from build123d import *

# Parameters (mm, degrees)
EXTRU_MINCE1_DEPTH      = 3
EXTRU_MINCE1_2_DEPTH    = 3
EXTRU_MINCE1_3_DEPTH    = 3
BOSS_EXTRU_1_DEPTH      = 0.25
BOSS_EXTRU_1_DEPTH_BACK = 1
ESQUISSE3_R             = 4.3
ESQUISSE3_R_2           = 0.05
ESQUISSE4_W             = 1.75
ESQUISSE4_H             = 3
EXTRU_MINCE2_DEPTH      = 45
CONG_1_R                = 0.2
ESQUISSE6_R             = 6.8
BOSS_EXTRU_2_DEPTH      = 1.3


# Read off the part's stored shape, not the designer's step: Extru.-Mince2
with BuildPart() as part:
    # Esquisse2 → Extru.-Mince1 (new body)
    with BuildSketch(Plane.XY):
        with BuildLine():
            ThreePointArc((0, 4.2), (2.89149518, 3.046187063), (4.194302481, 0.218693153))
            Line((4.194302481, 0.218693153), (0.049932172, 0.00260349))
            ThreePointArc((0.049932172, 0.00260349), (0.034422562, 0.036264132), (0, 0.05))
            Line((0, 0.05), (0, 4.2))
        make_face()
    extrude(amount=EXTRU_MINCE1_DEPTH)



with BuildPart() as body_2:
    # Esquisse2 → Extru.-Mince1 2 (new body)
    with BuildSketch(Plane.XY):
        with BuildLine():
            ThreePointArc((3.637306696, -2.1), (1.192327791, -4.027201813), (-1.907757414, -3.741719077))
            Line((-1.907757414, -3.741719077), (-0.022711398, -0.044544275))
            ThreePointArc((-0.022711398, -0.044544275), (0.014194378, -0.047942879), (0.04330127, -0.025))
            Line((0.04330127, -0.025), (3.637306696, -2.1))
        make_face()
    extrude(amount=EXTRU_MINCE1_2_DEPTH)


with BuildPart() as body_3:
    # Esquisse2 → Extru.-Mince1 3 (new body)
    with BuildSketch(Plane.XY):
        with BuildLine():
            ThreePointArc((-3.637306696, -2.1), (-4.083822971, 0.98101475), (-2.286545067, 3.523025923))
            Line((-2.286545067, 3.523025923), (-0.027220775, 0.041940785))
            ThreePointArc((-0.027220775, 0.041940785), (-0.04861694, 0.011678747), (-0.04330127, -0.025))
            Line((-0.04330127, -0.025), (-3.637306696, -2.1))
        make_face()
    extrude(amount=EXTRU_MINCE1_3_DEPTH)


with BuildPart() as part_1:
    add(part.part)

    add(body_2.part)  # Boss.-Extru.1 merges body 2

    add(body_3.part)  # Boss.-Extru.1 merges body 3
    # Esquisse3 → Boss.-Extru.1 (add, two sides: drawn at the far end of the back side and taken through both)
    # profile 1 of 2: a face of its own
    with BuildSketch(Plane.XY.offset(-BOSS_EXTRU_1_DEPTH_BACK)):
        Circle(ESQUISSE3_R)
        Circle(ESQUISSE3_R_2, mode=Mode.SUBTRACT)
    # profile 2 of 2: a face of its own
    with BuildSketch(Plane.XY.offset(-BOSS_EXTRU_1_DEPTH_BACK)):
        Circle(ESQUISSE3_R_2)
    extrude(amount=BOSS_EXTRU_1_DEPTH + BOSS_EXTRU_1_DEPTH_BACK)

    # Esquisse4 → Enlèvement de matière-Révolution1 (revolve, cut)
    with BuildSketch(Plane(origin=(0, 0, 0), x_dir=(0, 0, -1), z_dir=(1, 0, 0)), mode=Mode.PRIVATE) as enl_vement_de_mati_re_r_volution1_sk:
        with Locations((-1.625, 2.5)):
            Rectangle(ESQUISSE4_W, ESQUISSE4_H)
    revolve(enl_vement_de_mati_re_r_volution1_sk.sketch.rotate(Axis((0, 0, 0), (0, 0, 1)), 270), axis=Axis((0, 0, 0), (0, 0, 1)), mode=Mode.SUBTRACT)

    # Extru.-Mince2 outline → Extru.-Mince2 (add)
    with BuildSketch(Plane(origin=(0, 0, -1), x_dir=(-1, 0, 0), z_dir=(0, 0, -1))):
        Polygon((0.75, 1.03228644), (0.75, 3.7), (-0.75, 3.7), (-0.75, 1.03228644), (-3.287146365, 1.856655266), (-3.750671856, 0.430070492), (-1.213525492, -0.394298334), (-2.781568179, -2.55252394), (-1.568042688, -3.434201818), (0, -1.275976213), (1.568042688, -3.434201818), (2.781568179, -2.55252394), (1.213525492, -0.394298334), (3.750671856, 0.430070492), (3.287146365, 1.856655266), align=None)
    extrude(amount=EXTRU_MINCE2_DEPTH)

    # Congé1
    cong_1_edges = [part_1.edges().sort_by_distance(p)[0] for p in [
        (1.997546836, -1.473411137, -1),
        (2.018573182, 1.444470853, -1),
        (-2.482098674, 0.017886079, -1),
        (2.482098674, 0.017886079, -1),
        (3.518909111, 1.143362879, -1),
        (0.75, 2.36614322, -1),
        (0, 3.7, -1),
        (-2.018573182, 1.444470853, -1),
        (-3.51890911, 1.143362879, -1),
        (-1.997546836, -1.473411137, -1),
        (-2.174805433, -2.993362879, -1),
        (0.784021344, -2.355089015, -1),
        (2.174805433, -2.993362879, -1),
        (-0.75, 2.36614322, -1),
        (-0.784021344, -2.355089015, -1),
    ]]
    fillet(cong_1_edges, radius=CONG_1_R)

    # Esquisse6 → Boss.-Extru.2 (add)
    with BuildSketch(Plane(origin=(0, 0, -46), x_dir=(-1, 0, 0), z_dir=(0, 0, -1))):
        Circle(ESQUISSE6_R)
    extrude(amount=BOSS_EXTRU_2_DEPTH)


solid = part_1.part
The model under review builds one solid part; all positions refer to its coordinate system, in mm. A direction names the side the tool comes from. Round coordinates to 2 decimals unless told otherwise and drop trailing zeros. Write each loop counter-clockwise with the first axis right and the second up, starting at its lowest first coordinate (ties: lowest second). Pieces come first, ordered by that corner, then holes. Notation, with made-up numbers: (22.25, -18) -> (60.25, -18) arc R31 cw to (60.25, 10) -> close; hole circle Ø6 at (20.25, 43). An arc over 180 degrees is marked (long way). Answer as a JSON object with one key per item and string values.
1. To check wall thickness, follow line 1 along Z through (x, y) = (-5, -1.75); line 2 along X through (y, z) = (2.25, -33.5); line 3 along Y through (x, z) = (-2.25, -5). State the ranges of each line that lie inside material, in increasing order.
Results found:
{"line 1": "z = -47.3 to -46", "line 2": "x = -0.75 to 0.75", "line 3": "y = -2.94 to -1.82, -0.06 to 1.52"}
2. The part is to be moulded in two halves that separate along Z. For faces 1 (the face through (-3, 1, 3)), 2 (the face through (2.859, 3.077, 1.606)), 3 (the face through (2.114, 1.539, -1.057)), say which applies: pulls with the +Z half, pulls with the -Z half, needs draft (parallel to the pull), parting line crosses it, or undercut.
Results found:
{"face 1": "pulls with the +Z half", "face 2": "needs draft", "face 3": "undercut"}
3. We need section A-A on z = -9.5. State the section outline as (x, y) points, and give its area (3 significant figures).
Results found:
{"outline": "(-3.75, 0.43) -> (-1.21, -0.39) -> (-2.78, -2.55) -> (-1.57, -3.43) -> (0, -1.28) -> (1.57, -3.43) -> (2.78, -2.55) -> (1.21, -0.39) -> (3.75, 0.43) -> (3.29, 1.86) -> (0.75, 1.03) -> (0.75, 3.7) -> (-0.75, 3.7) -> (-0.75, 1.03) -> (-3.29, 1.86) -> close", "area": "23.9 mm^2"}
4. Machinability: for faces 4 (the face through (0.75, 2, -23)), 5 (the face through (-2.09, -1.5, -1.06)), 6 (the face through (2.5, 0.024, -23.286)), 7 (the face through (-2.22, -3.03, -1.06)), which of the approach directions +Z, -Z, +X, -X, +Y, -Y give a long, thin tool a straight path to every point of the face, cutting with its end or side? Answer none if there is none.
Results found:
{"face 4": "+Y", "face 5": "-X", "face 6": "+X", "face 7": "-X, -Y"}
5. Clearance check with flat-ended pins moving along their axes: pin 1 (1.6 mm diameter, centred on x = -0.5, z = -28.5, fed in from +Y); pin 2 (6 mm diameter, centred on y = -2, z = -20.5, fed in from -X); pin 3 (1.4 mm diameter, centred on y = 1, z = 2, fed in from -X). State where each tip first meets the part, or that it passes through.
Results found:
{"pin 1": "stops at y = 3.7", "pin 2": "stops at x = -3.75", "pin 3": "stops at x = -4.19"}
6. We need section B-B on y = 5. State the section outline as (x, z) points, and give its area (3 significant figures).
Results found:
{"outline": "(-4.61, -47.3) -> (4.61, -47.3) -> (4.61, -46) -> (-4.61, -46) -> close", "area": "12.0 mm^2"}
